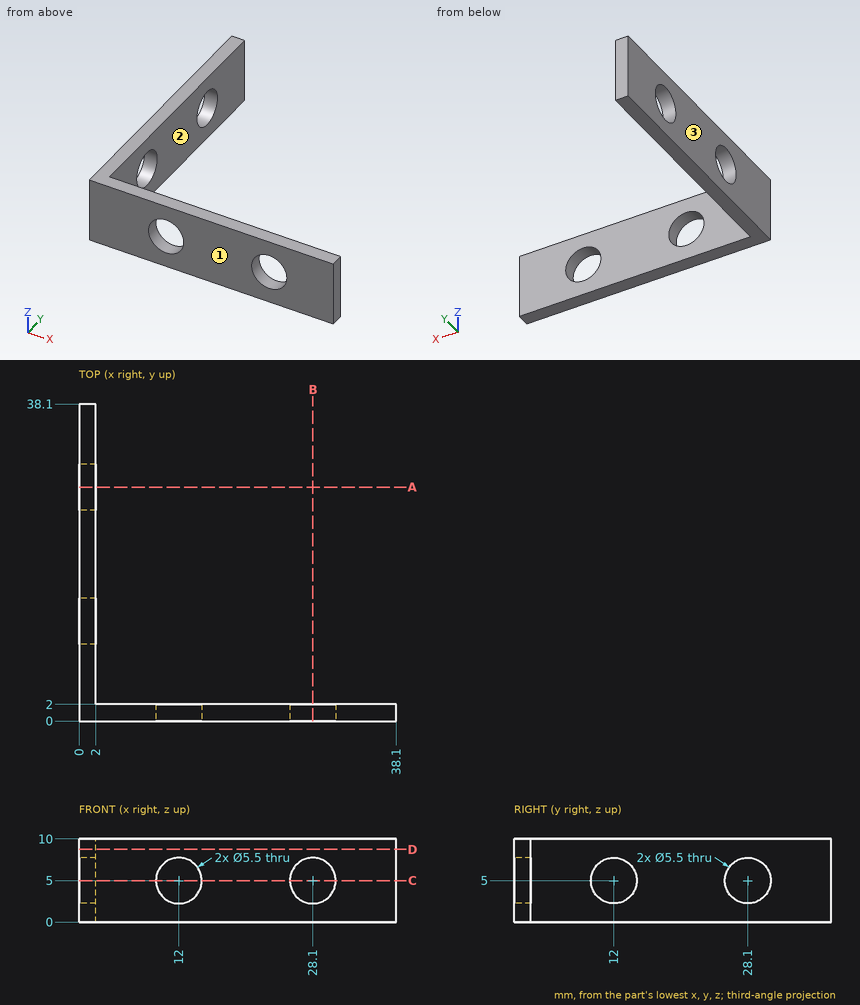
Geometry: see drawing. Coordinates: mm, zero at the bounding-box minimum. Round coordinates to 2 decimals unless told otherwise and drop trailing zeros. Write each loop counter-clockwise with the first axis right and the second up, starting at its lowest first coordinate (ties: lowest second). Pieces come first, ordered by that corner, then holes. Notation, with made-up numbers: (40.5, -14.5) - (53.5, -14.5) arc R20 cw to (53.5, -1.5) - close; hole circle Ø5 at (3, -29.75). An arc over 180 degrees is marked (long way). Use CSV: the item, a comma, the result in double quotes. Start each with the question number.
(1) First-contact query: pin 1 Ø4 at (y, z) = (27, 4.5) entering from +X; pin 2 Ø10 at (x, y) = (19.5, 8.5) entering from -Z; pin 3 Ø3 at (y, z) = (10.5, 2.5) entering from -X; pin 4 Ø2 at (x, z) = (22.5, 8) entering from +Y. Flat tips, straight axial feed; report the tip coordinate or a pass-through.
(2) Mould query, pull axis X, two halves, no side actions, for the marked faces 1, 2 and 3. Classes: pulls with the +X half, pulls with the -X half, needs draft (parallel to the pull), parting line crosses it, or undercut.
(3) Material intervals for probe 1 along X at (y, z) = (0.95, 5); probe 2 along Z at (x, y) = (28, 1); probe 3 along Y at (x, z) = (28.5, 1.5), sorted ascending. Write a range as [from, to].
(4) Cut plane C-C, the plane z = 5. Return loops of the section in (x, y), and give its area (3 significant figures).
(5) Cut plane D-D, the plane z = 8.75. Return loops of the section in (x, y), and give its area (3 significant figures).
(6) Cut plane A-A, the plane y = 28.1. Return loops of the section in (x, z).
Geometry says:
1,pin 1,"x = 2"
1,pin 2,"through"
1,pin 3,"x = 0"
1,pin 4,"y = 2"
2,face 1,"needs draft"
2,face 2,"pulls with the +X half"
2,face 3,"pulls with the -X half"
3,probe 1,"[0, 9.25], [14.75, 25.35], [30.85, 38.1]"
3,probe 2,"[0, 2.25], [7.75, 10]"
3,probe 3,"[0, 2]"
4,outline,"(0, 0) - (9.25, 0) - (9.25, 2) - (2, 2) - (2, 9.25) - (0, 9.25) - close; (0, 14.75) - (2, 14.75) - (2, 25.35) - (0, 25.35) - close; (0, 30.85) - (2, 30.85) - (2, 38.1) - (0, 38.1) - close; (14.75, 0) - (25.35, 0) - (25.35, 2) - (14.75, 2) - close; (30.85, 0) - (38.1, 0) - (38.1, 2) - (30.85, 2) - close"
4,area,"104 mm²"
5,outline,"(0, 0) - (38.1, 0) - (38.1, 2) - (2, 2) - (2, 38.1) - (0, 38.1) - close"
5,area,"148 mm²"
6,outline,"(0, 0) - (2, 0) - (2, 2.25) - (0, 2.25) - close; (0, 7.75) - (2, 7.75) - (2, 10) - (0, 10) - close"
